Geometry check sheet. Reference: the model listing, model coordinates, mm. A direction names the side the tool comes from. Round coordinates to 2 decimals unless told otherwise and drop trailing zeros. Order: outer loops, then holes, each group sorted by start corner. A loop starts at its lowest first (then second) coordinate and runs counter-clockwise, first axis right, second up.
```python
from build123d import *

# Parameters (mm, degrees)
F0_W     = 59.7408
F0_H     = 10.16
F1_DEPTH = 2.032
F4_DEPTH = 10.16
F6_DEPTH = 10.161


with BuildPart() as f1:
    # F0 (on Top) → F1 (new body)
    with BuildSketch(Plane.XY):
        with Locations((10.114113, -35.470716)):
            Rectangle(F0_W, F0_H)
        with BuildLine():
            ThreePointArc((39.984513, -40.550716), (45.064513, -35.470716), (39.984513, -30.390716))
            Line((39.984513, -30.390716), (39.984513, -40.550716))
        make_face()
    extrude(amount=F1_DEPTH)

    # F3 (on face) → F4 (join)
    with BuildSketch(Plane.XZ.offset(40.550716)):
        Polygon((31.856513, 2.032), (39.984513, 2.032), (31.856513, 5.632), align=None)
    extrude(amount=-F4_DEPTH)

    # F5 (on face) → F6 (cut, through all)
    with BuildSketch(Plane.XZ.offset(40.550716)):
        Polygon((33.856513, 2.032), (31.856513, 4.032), (31.856513, 2.032), align=None)
    extrude(amount=-F6_DEPTH, mode=Mode.SUBTRACT)


solid = f1.part
```
(1) Draft check along Z on faces 4 (the flat face through (12, -35, 0)), 5 (the flat face through (35.977, -35.542, 3.807)), 6 (the flat face through (32.87, -35.54, 3.02)). Enter one of: released by +Z, released by -Z, zero draft, split by the parting line, or undercut.
Returned:
face 4: released by -Z
face 5: released by +Z
face 6: undercut
(2) Sectioned sample at A-A, the plane y = -39.5. Record the cut outline in (x, z).
Returned:
outline: (-19.76, 0) - (43.08, 0) - (43.08, 2.03) - (39.98, 2.03) - (31.86, 5.63) - (31.86, 4.03) - (33.86, 2.03) - (-19.76, 2.03) - close
(3) Sectioned sample at B-B, the plane x = 9.5. Record the cut outline in (y, z).
Returned:
outline: (-40.55, 0) - (-30.39, 0) - (-30.39, 2.03) - (-40.55, 2.03) - close
(4) Depth check by flat-ended pin: P1, Ø0.8, axis at y = -34, z = 5, coming from the -X side; P2, Ø6, axis at x = -4.5, y = -37, coming from the +Z side. Enter the tip coordinate at first touch or a pass-through.
Returned:
P1: stops at x = 31.86
P2: stops at z = 2.03
(5) Sectioned sample at C-C, the plane z = 1.4. Record the cut outline in (x, y), and give its area (3 significant figures).
Returned:
outline: (-19.76, -40.55) - (39.98, -40.55) arc R5.08 ccw to (39.98, -30.39) - (-19.76, -30.39) - close
area: 648 mm2
(6) Set-up check for faces 1 (the flat face through (42, -35, 2.032)), 2 (the flat face through (-19.756, -36, 1)), 3 (the flat face through (31.857, -36, 5)): record each of +Z, -Z, +X, -X, +Y, -Y from which the full face is reachable in a straight line by a thin tool's end or side.
Returned:
face 1: +Z, +X, +Y, -Y
face 2: +Z, -Z, -X, +Y, -Y
face 3: +Z, -X, +Y, -Y
(7) Material ranges on line 1 (Z direction, x = 35.5, y = -37.75); line 2 (Z direction, x = 28, y = -36.25); line 3 (X direction, y = -35.25, z = 4.1), recorded low to high.
Returned:
line 1: z = 0 to 4.02
line 2: z = 0 to 2.03
line 3: x = 31.86 to 35.32
(8) Sectioned sample at D-D, the plane y = -35.25. Record the cut outline in (x, z), and give its area (3 significant figures).
Returned:
outline: (-19.76, 0) - (45.06, 0) - (45.06, 2.03) - (39.98, 2.03) - (31.86, 5.63) - (31.86, 4.03) - (33.86, 2.03) - (-19.76, 2.03) - close
area: 144 mm2
